Autodesk Inventor part; units mm, degrees
ref_plane "YZ Plane" through (0, 0, 0) normal (1, 0, 0) x (0, 1, 0)
ref_plane "XZ Plane" through (0, 0, 0) normal (0, 1, 0) x (-1, 0, 0)
ref_plane "XY Plane" through (0, 0, 0) normal (0, 0, 1) x (1, 0, 0)
sketch "Sketch1" plane through (0, 0, 0) normal (0, 0, 1) x (1, 0, 0)
  line L0 (0, 0) -> (2.5, 0)
  line L1 (2.5, 0) -> (2.5, -6.731)
  line L2 (2.5, -6.731) -> (17.5, -6.731)
  line L3 (17.5, -6.731) -> (17.5, 0)
  line L4 (17.5, 0) -> (20, 0)
  line L5 (20, 0) -> (20, 18.731)
  line L6 (20, 18.731) -> (12.5, 18.731)
  line L7 (12.5, 18.731) -> (12.5, 12)
  line L8 (12.5, 12) -> (7.5, 12)
  line L9 (7.5, 12) -> (7.5, 18.731)
  line L10 (7.5, 18.731) -> (0, 18.731)
  line L11 (0, 18.731) -> (0, 0)
  dimension "d0" = 15
  dimension "d1" = 20
  dimension "d3" = 6.731
  dimension "d4" = 5
  dimension "d5" = 12
extrude "Extrusion1" add sketch "Sketch1" along normal blind 6.731
sketch "Sketch2" plane through (0, 0, 0) normal (0, 0, -1) x (-1, 0, 0)
  line L0 (0, 0) -> (-2.5, 0)
  circle A0 centre (-5, 3) radius 1.588
  circle A1 centre (-5, 9) radius 1.588
  line L1 (-12.5, 12) -> (-7.5, 12)
  line L2 (-2.5, 0) -> (-2.5, -6.731)
  line L3 (-10, 12) -> (-10, 9.3655) construction
  dimension "d8" = 6
  dimension "d9" = 3.176
  dimension "d10" = 3
  dimension "d22" = 5
extrude "Extrusion2" cut sketch "Sketch2" against normal up to next
fillet "Fillet1" radius 5 2 edges at (0, 18.731, 3.3655) (20, 18.731, 3.3655)
sketch "Sketch3" plane through (0, 0, 6.731) normal (0, 0, 1) x (1, 0, 0)
  circle A0 centre (5, 3) radius 1.588
  circle A1 centre (5, 9) radius 1.588
  line L0 (8.4641, 9) -> (6.7321, 6)
  line L1 (6.7321, 6) -> (3.2679, 6)
  line L2 (3.2679, 6) -> (1.5359, 9)
  line L3 (1.5359, 9) -> (3.2679, 12)
  line L4 (3.2679, 12) -> (6.7321, 12)
  line L5 (6.7321, 12) -> (8.4641, 9)
  line L6 (8.4641, 3) -> (6.7321, 0)
  line L7 (6.7321, 0) -> (3.2679, 0)
  line L8 (3.2679, 0) -> (1.5359, 3)
  line L9 (1.5359, 3) -> (3.2679, 6)
  line L10 (3.2679, 6) -> (6.7321, 6)
  line L11 (6.7321, 6) -> (8.4641, 3)
  dimension "d14" = 6
extrude "Extrusion3" cut sketch "Sketch3" against normal blind 3
sketch "Sketch4" plane through (0, 0, 6.731) normal (0, 0, 1) x (1, 0, 0)
  circle A0 centre (7.5, 13.5875) radius 1.5875
  circle A1 centre (12.5, 13.5875) radius 1.5875
  line L0 (12.5, 18.731) -> (12.5, 12)
  line L1 (0, 0) -> (2.5, 0)
  line L2 (2.5, 0) -> (2.5, -6.731)
  line L3 (17.5, -6.731) -> (17.5, 0)
  line L4 (17.5, 0) -> (20, 0)
  arc A2 (2.5, -3.175) -> (2.5, 0) centre (2.5, -1.5875) ccw
  arc A3 (17.5, 0) -> (17.5, -3.175) centre (17.5, -1.5875) ccw
  dimension "d17" = 3.175
extrude "Extrusion4" cut sketch "Sketch4" against normal up to next
equation "\"d3\" = THICKB"
equation "\"d6\" = THICKB"
equation "\"THICKA\" = 3.175"
equation "\"THICKB\" = 6.731"
equation "\"THICKC\" = 12.7"
equation "\"THICKPLY\" = 5"
equation "\"MAGDIA\" = 9.5"
equation "\"BALLDIA\" = 12"
properties part number "Carriage_Joint_Boltblock"
The model under review builds one solid part; all positions refer to its coordinate system, in mm. A direction names the side the tool comes from. Round coordinates to 2 decimals unless told otherwise and drop trailing zeros. Order: outer loops, then holes, each group sorted by start corner. A loop starts at its lowest first (then second) coordinate and runs counter-clockwise, first axis right, second up. Notation, with made-up numbers: (73, 64) -> (124, 64) arc R28 ccw to (124, 90) -> close; hole circle Ø4 at (89.25, 57.25). An arc over 180 degrees is marked (long way). Return JSON: item names as keys, results as strings.
1. Take a section at A-A (z = 6). Write out the cut boundary in (x, y) (1 decimal).
Answer block:
{"outline": "(0, 0) -> (2.5, 0) arc R1.6 cw to (2.5, -3.2) -> (2.5, -6.7) -> (17.5, -6.7) -> (17.5, -3.2) arc R1.6 cw to (17.5, 0) -> (20, 0) -> (20, 13.7) arc R5 ccw to (15, 18.7) -> (12.5, 18.7) -> (12.5, 15.2) arc R1.6 cw to (12.5, 12) -> (7.5, 12) arc R1.6 cw to (7.5, 15.2) -> (7.5, 18.7) -> (5, 18.7) arc R5 ccw to (0, 13.7) -> close; hole (1.5, 3) -> (3.3, 0) -> (6.7, 0) -> (8.5, 3) -> (6.7, 6) -> (8.5, 9) -> (6.7, 12) -> (3.3, 12) -> (1.5, 9) -> (3.3, 6) -> close"}
2. Take a section at C-C (z = 2.75). Write out the cut boundary in (x, y) (1 decimal), then the cut area to 3 significant figures.
Answer block:
{"outline": "(0, 0) -> (2.5, 0) arc R1.6 cw to (2.5, -3.2) -> (2.5, -6.7) -> (17.5, -6.7) -> (17.5, -3.2) arc R1.6 cw to (17.5, 0) -> (20, 0) -> (20, 13.7) arc R5 ccw to (15, 18.7) -> (12.5, 18.7) -> (12.5, 15.2) arc R1.6 cw to (12.5, 12) -> (7.5, 12) arc R1.6 cw to (7.5, 15.2) -> (7.5, 18.7) -> (5, 18.7) arc R5 ccw to (0, 13.7) -> close; hole circle Ø3.2 at (5, 3); hole circle Ø3.2 at (5, 9)", "area": "400 mm²"}
3. For faces 1 (the face through (5, 12, 5)), 2 (the face through (2.5, -5, 3)), 3 (the face through (5.913, 13.622, 3.413)), list the 3-axis set-ups (+Z, -Z, +X, -X, +Y, -Y) from which the entire face can be reached by the end or side of a thin tool; tool diameter is ignored.
Answer block:
{"face 1": "+Z", "face 2": "+Z, -Z, -X, -Y", "face 3": "+Z, -Z"}
4. Take a section at D-D (y = 2.25). Write out the cut boundary in (x, z), then the cut area to 3 significant figures.
Answer block:
{"outline": "(0, 0) -> (3.6, 0) -> (3.6, 3.73) -> (1.97, 3.73) -> (1.97, 6.73) -> (0, 6.73) -> close; (6.4, 0) -> (20, 0) -> (20, 6.73) -> (8.03, 6.73) -> (8.03, 3.73) -> (6.4, 3.73) -> close", "area": "106 mm²"}
5. Take a section at B-B (x = 13.25). Write out the cut boundary in (y, z).
Answer block:
{"outline": "(-6.73, 0) -> (12.19, 0) -> (12.19, 6.73) -> (-6.73, 6.73) -> close; (14.99, 0) -> (18.73, 0) -> (18.73, 6.73) -> (14.99, 6.73) -> close"}
6. The part is to be moulded in two halves that separate along Y. For faces 4 (the face through (1.5, 17.3, 3.4)), 5 (the face through (5, 0, 5)), 6 (the face through (1, 0, 3)), 7 (the face through (12.5, 17, 3)), say which applies: +Y half, -Y half, draft (parallel to the pull), parting line (faces both ways), or undercut.
Answer block:
{"face 4": "+Y half", "face 5": "undercut", "face 6": "-Y half", "face 7": "draft"}
7. Insertion check: P1, Ø2, axis at x = 9, y = -0.5, coming from the -Z side; P2, Ø0.8, axis at x = 18, z = 2, coming from the -Y side; P3, Ø4, axis at y = 16.5, z = 3, coming from the +X side; P4, Ø1.5, axis at x = 10.5, z = 4.5, coming from the +Y side. Each pin has a flat end and moves straight along its axis. Give the tip position at first contact, or say it passes through.
Answer block:
{"P1": "stops at z = 0", "P2": "stops at y = 0", "P3": "stops at x = 19.94", "P4": "stops at y = 12"}
8. For L1, parallel to Y at x = 5, z = 1.7; L2, parallel to X at y = 3, z = 1; L3, parallel to Y at x = 12, z = 5.25, list the stretches that pass through material, from the lowest coordinate up. Write a range as [from, to].
Answer block:
{"L1": "y = [-6.73, 1.41], [4.59, 7.41], [10.59, 18.73]", "L2": "x = [0, 3.41], [6.59, 20]", "L3": "y = [-6.73, 12]"}
